from build123d import *

# Parameters (mm, degrees)
SKETCH_1_W      = 36
SKETCH_1_H      = 27
EXTRUDE_1_DEPTH = 74
SKETCH_2_R      = 2
SKETCH_7_R      = 2


with BuildPart() as part:
    # Эскиз1 → Бобышка-Вытянуть1 (new body)
    with BuildSketch(Plane(origin=(0, 0, 0), x_dir=(1, 0, 0), z_dir=(0, 1, 0))):
        Rectangle(SKETCH_1_W, SKETCH_1_H)
    extrude(amount=EXTRUDE_1_DEPTH)

    # По траектории1: sweep along a path in Эскиз4
    with BuildLine() as sweep_1_path:  # in the path sketch's own coordinates; laid on its plane below (add() does not lay a ready-made edge on the line's plane)
        add(Edge.make_bspline(
            [(-18, -66.076411234), (-23.742943234, -66.28318966), (-23.404198894, -83.547219803), (-23, -87.819533928)],
            knots=[0, 0, 0, 0, 1, 1, 1, 1], degree=3))
    # Эскиз2 → По траектории1 (sweep)
    with BuildSketch(Plane(origin=(18, 0, 0), x_dir=(0, 0, -1), z_dir=(1, 0, 0))):
        with Locations((-9.5, 72)):
            Circle(SKETCH_2_R)
    sweep(path=Plane(origin=(0, 8.81081368, 28.818872995), x_dir=(-1, 0, 0), z_dir=(0, 0.2923717047227373, 0.9563047559630353)) * sweep_1_path.line)

    # По траектории2: sweep along a path in Эскиз6
    with BuildLine() as sweep_2_path:  # in the path sketch's own coordinates; laid on its plane below (add() does not lay a ready-made edge on the line's plane)
        add(Edge.make_bspline(
            [(-18, 66.076411234), (-21.87269918, 66.293847573), (-23.822441066, 75.687463782), (-23, 87.819533928)],
            knots=[0, 0, 0, 0, 1, 1, 1, 1], degree=3))
    # Эскиз7 → По траектории2 (sweep)
    with BuildSketch(Plane(origin=(18, 0, 0), x_dir=(0, 0, -1), z_dir=(1, 0, 0))):
        with Locations((9.5, 72)):
            Circle(SKETCH_7_R)
    sweep(path=Plane(origin=(0, 8.81081368, -28.818872995), x_dir=(-1, 0, 0), z_dir=(0, 0.2923717047227373, -0.9563047559630353)) * sweep_2_path.line)


solid = part.part
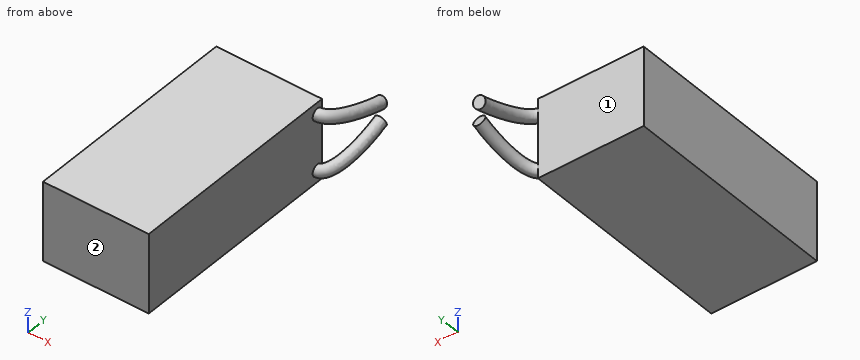
The model under review builds one solid part; all positions refer to its coordinate system, in mm. Face numbers are marked on the shaded views. A direction names the side the tool comes from. Give positions to 0.01 mm unless a question says otherwise; leave off trailing zeros. Order: outer loops, then holes, each group sorted by start corner. A loop starts at its lowest first (then second) coordinate and runs counter-clockwise, first axis right, second up. Notation, with made-up numbers: (48, 16.25) -> (96, 16.25) arc R18 ccw to (96, 40.25) -> close; hole circle Ø4 at (15.5, -4). An arc over 180 degrees is marked (long way). Write item = value, one per line. Start each with the question number.
(1) Tool access review of the marked faces 1 and 2: name each direction out of +Z, -Z, +X, -X, +Y, -Y from which nothing blocks a thin tool from reaching the whole face with its end or side.
(2) Take a section at A-A (x = -7). Write out the cut boundary in (y, z), plus the area to 3 significant figures.
(3) For pin 1 Ø6 at (y, z) = (11.5, -4) entering from +X; pin 2 Ø12 at (x, z) = (12.5, 0.5) entering from +Y, all flat-tipped, find the tip position at first contact; note any pin that passes through.
(4) Take a section at B-B (y = 63.5). Write out the cut boundary in (x, z).
(5) For L1, parallel to Y at x = 13.5, z = 11.75; L2, parallel to X at y = 13, z = 8; L3, parallel to X at y = 81.5, z = 7.25, list the stretches that pass through material, from the lowest coordinate up. Write a range as from..to.
Returned:
q1.face_1 = +Z, -Z, -X, +Y
q1.face_2 = +Z, -Z, +X, -X, -Y
q2.outline = (0, -13.5) -> (74, -13.5) -> (74, 13.5) -> (0, 13.5) -> close
q2.area = 2,000 mm²
q3.pin_1 = 18
q3.pin_2 = 74
q4.outline = (-18, -13.5) -> (18, -13.5) -> (18, 13.5) -> (-18, 13.5) -> close
q5.L1 = 0..74
q5.L2 = -18..18
q5.L3 = 20.94..24.76
